Could you check a few things on this model? Use its own coordinates, in mm. A direction names the side the tool comes from. Give positions to 0.01 mm unless a question says otherwise; leave off trailing zeros. Order: outer loops, then holes, each group sorted by start corner. A loop starts at its lowest first (then second) coordinate and runs counter-clockwise, first axis right, second up. Notation, with made-up numbers: M 37,-2 L 86,-2 A15 ccw 86,16 Z; hole C 54.5,-36 d7. An arc over 180 degrees is marked long. Answer in a Markdown table with one row per item. Add a question column.
```python
from build123d import *

# Parameters (mm, degrees)
EXTRUDE_1_DEPTH     = 30
SKETCH_2_W          = 15
SKETCH_2_H          = 5
EXTRUDE_2_DEPTH     = 30
EXTRUDE_3_DEPTH     = 30
CUT_EXTRUDE_1_REACH = 111.107
SKETCH_6_R          = 1.7
SKETCH_7_W          = 60
SKETCH_7_H          = 60
EXTRUDE_4_DEPTH     = 4


# Read off the part's stored shape, not the designer's step: M3 すきま穴1, M3 すきま穴2
with BuildPart() as part:
    # ｽｹｯﾁ1 → ﾎﾞｽ - 押し出し1 (new body)
    with BuildSketch(Plane.XY):
        with BuildLine():
            Line((-57.15, 0), (-61.15, 0))
            ThreePointArc((-61.15, 0), (0, 61.15), (61.15, 0))
            Line((61.15, 0), (57.15, 0))
            ThreePointArc((57.15, 0), (0, 57.15), (-57.15, 0))
        make_face()
    extrude(amount=EXTRUDE_1_DEPTH)

    # ｽｹｯﾁ2 → ﾎﾞｽ - 押し出し2 (add)
    with BuildSketch(Plane.XY.offset(30)):
        with Locations((-64.65, 2.5)):
            Rectangle(SKETCH_2_W, SKETCH_2_H)
        with Locations((64.65, 2.5)):
            Rectangle(SKETCH_2_W, SKETCH_2_H)
    extrude(amount=-EXTRUDE_2_DEPTH)

    # M3 すきま穴1 outline → M3 すきま穴1 (revolve, cut)
    with BuildSketch(Plane(origin=(66.547620908, 0, 25), x_dir=(1, 0, 0), z_dir=(0, 0, 1))):
        Polygon((0, 0), (1.7, 0), (1.7, 4.97124079), (1.725, 5), (0, 5), align=None)
    revolve(axis=Axis((66.547620908, 0, 25), (0, 1, 0)), mode=Mode.SUBTRACT)

    # Hole Wizard M3 _1 2 outline → Hole Wizard M3 _1 2 (revolve, cut)
    with BuildSketch(Plane(origin=(66.547620908, 0, 5), x_dir=(1, 0, 0), z_dir=(0, 0, 1))):
        Polygon((0, 0), (1.7, 0), (1.7, 4.97124079), (1.725, 5), (0, 5), align=None)
    revolve(axis=Axis((66.547620908, 0, 5), (0, 1, 0)), mode=Mode.SUBTRACT)

    # Hole Wizard M3 _1 3 outline → Hole Wizard M3 _1 3 (revolve, cut)
    with BuildSketch(Plane(origin=(-66.547620908, 0, 25), x_dir=(1, 0, 0), z_dir=(0, 0, 1))):
        Polygon((0, 0), (1.7, 0), (1.7, 4.97124079), (1.725, 5), (0, 5), align=None)
    revolve(axis=Axis((-66.547620908, 0, 25), (0, 1, 0)), mode=Mode.SUBTRACT)

    # Hole Wizard M3 _1 4 outline → Hole Wizard M3 _1 4 (revolve, cut)
    with BuildSketch(Plane(origin=(-66.547620908, 0, 5), x_dir=(1, 0, 0), z_dir=(0, 0, 1))):
        Polygon((0, 0), (1.7, 0), (1.7, 4.97124079), (1.725, 5), (0, 5), align=None)
    revolve(axis=Axis((-66.547620908, 0, 5), (0, 1, 0)), mode=Mode.SUBTRACT)

    # ｽｹｯﾁ5 → ﾎﾞｽ - 押し出し3 (add)
    with BuildSketch(Plane.XY.offset(30)):
        Polygon((-15, 57.15), (15, 57.15), (15, 72.15), (30, 72.15), (30, 76.15), (-30, 76.15), (-30, 72.15), (-15, 72.15), align=None)
    extrude(amount=-EXTRUDE_3_DEPTH)

    # ｽｹｯﾁ6 → ｶｯﾄ - 押し出し1 (cut, up to next)
    with BuildSketch(Plane(origin=(0, 76.15, 0), x_dir=(1, 0, 0), z_dir=(0, 1, 0)), mode=Mode.PRIVATE) as cut_extrude_1_sk1:
        with Locations(Location((-25, -15, 0), (0, 0, 180))):
            Circle(SKETCH_6_R)
    cut_extrude_1_tool1 = extrude(cut_extrude_1_sk1.sketch, amount=-CUT_EXTRUDE_1_REACH, mode=Mode.PRIVATE) & part.part
    # ｽｹｯﾁ6 → ｶｯﾄ - 押し出し1 (cut, up to next)
    with BuildSketch(Plane(origin=(0, 76.15, 0), x_dir=(1, 0, 0), z_dir=(0, 1, 0)), mode=Mode.PRIVATE) as cut_extrude_1_sk2:
        with Locations(Location((25, -15, 0), (0, 0, 180))):
            Circle(SKETCH_6_R)
    cut_extrude_1_tool2 = extrude(cut_extrude_1_sk2.sketch, amount=-CUT_EXTRUDE_1_REACH, mode=Mode.PRIVATE) & part.part
    add(cut_extrude_1_tool1.solids().sort_by_distance((-25, 76.15, 15))[0], mode=Mode.SUBTRACT)
    add(cut_extrude_1_tool2.solids().sort_by_distance((25, 76.15, 15))[0], mode=Mode.SUBTRACT)

    # ｽｹｯﾁ7 → ﾎﾞｽ - 押し出し4 (add)
    with BuildSketch(Plane(origin=(0, 76.15, 0), x_dir=(1, 0, 0), z_dir=(0, 1, 0))):
        with Locations((0, -60)):
            Rectangle(SKETCH_7_W, SKETCH_7_H)
    extrude(amount=-EXTRUDE_4_DEPTH)

    # M3 すきま穴2 outline → M3 すきま穴2 (revolve, cut)
    with BuildSketch(Plane(origin=(-17.5, 0, 85), x_dir=(1, 0, 0), z_dir=(0, 0, 1))):
        Polygon((0, 72.15), (1.7, 72.15), (1.7, 76.12124079), (1.725, 76.15), (0, 76.15), align=None)
    revolve(axis=Axis((-17.5, 0, 85), (0, 1, 0)), mode=Mode.SUBTRACT)

    # Hole Wizard M3 _2 2 outline → Hole Wizard M3 _2 2 (revolve, cut)
    with BuildSketch(Plane(origin=(17.5, 0, 85), x_dir=(1, 0, 0), z_dir=(0, 0, 1))):
        Polygon((0, 72.15), (1.7, 72.15), (1.7, 76.12124079), (1.725, 76.15), (0, 76.15), align=None)
    revolve(axis=Axis((17.5, 0, 85), (0, 1, 0)), mode=Mode.SUBTRACT)


solid = part.part
```
1. Thinking about a two-plate mould opening in Z: for faces 6 (the flat face through (0, 74, 90)), 7 (the flat face through (-72.15, 2, 15)), 8 (the cylindrical face through (65.295, 2.52, 23.851)), which applies, pulls with the +Z half, pulls with the -Z half, needs draft (parallel to the pull), parting line crosses it, or undercut?
2. For faces 1 (the cylindrical face through (1.257, 57.136, 14.79)), 2 (the flat face through (30, 74, 46)), 3 (the cylindrical face through (23.43, 74.18, 14.35)), 4 (the flat face through (-30, 74, 46)), 5 (the cylindrical face through (46.33, 39.91, 14.79)), which set-ups out of +Z, -Z, +X, -X, +Y, -Y let a thin tool reach every point of the face, with its end or its side?
3. Suppose I cut it at B-B on y = 35.5. List the corners of the cut face in (x, z) for me.
4. Suppose I cut it at D-D on z = 85. List the corners of the cut face in (x, y) for me (3 decimals).
5. Will these pins go through, and if not, where does the flat tip stop? P1, Ø2, axis at x = 66.55, z = 25, coming from the +Y side; P2, Ø4.5, axis at y = 73.5, z = 24.5, coming from the +X side; P3, Ø18, axis at x = -5, z = 59.5, coming from the -Y side; P4, Ø8, axis at y = 10, z = 28.5, coming from the -X side.
6. Suppose I cut it at A-A on z = 25. Count the separate pieces of the cut face and the enclosed holes in it, plus the area to 3 significant figures.
7. If I drill on line 1 along Z through (x, y) = (25, 73); line 2 along X through (y, z) = (13.5, 21); line 3 along Y through (x, z) = (-27, 47), over which ranges is the centre line in solid material (lowest first)? Write a range as [from, to].
8. Suppose I cut it at C-C on x = 17.5. List the corners of the cut face in (y, z) for me (3 decimals).
Findings below:
| question | item | result |
|---|---|---|
| 1 | face 6 | pulls with the +Z half |
| 1 | face 7 | needs draft |
| 1 | face 8 | undercut |
| 2 | face 1 | +Z, -Z, -Y |
| 2 | face 2 | +Z, -Z, +X, +Y |
| 2 | face 3 | +Y |
| 2 | face 4 | +Z, -Z, -X, +Y |
| 2 | face 5 | +Z, -Z, +X |
| 3 | outline | M -49.79,0 L -44.79,0 L -44.79,30 L -49.79,30 Z; M 44.79,0 L 49.79,0 L 49.79,30 L 44.79,30 Z |
| 4 | outline | M -30,72.15 L -19.2,72.15 L -19.2,76.121 L -19.225,76.15 L -30,76.15 Z; M -15.8,72.15 L 15.8,72.15 L 15.8,76.121 L 15.775,76.15 L -15.775,76.15 L -15.8,76.121 Z; M 19.2,72.15 L 30,72.15 L 30,76.15 L 19.225,76.15 L 19.2,76.121 Z |
| 5 | P1 | through |
| 5 | P2 | x = 30 |
| 5 | P3 | y = 72.15 |
| 5 | P4 | x = -60.85 |
| 6 | separate pieces | 3 |
| 6 | enclosed holes | 0 |
| 6 | area | 1,410 mm2 |
| 7 | line 1 | [0, 13.3], [16.7, 90] |
| 7 | line 2 | [-59.64, -55.53], [55.53, 59.64] |
| 7 | line 3 | [72.15, 76.15] |
| 8 | outline | M 54.405,0 L 58.592,0 L 58.592,30 L 54.405,30 Z; M 72.15,0 L 76.15,0 L 76.15,83.275 L 76.121,83.3 L 72.15,83.3 Z; M 72.15,86.7 L 76.121,86.7 L 76.15,86.725 L 76.15,90 L 72.15,90 Z |
